Read the model definition and answer for the solid it produces. Units are mm, in the model's axes. Face numbers are marked on the shaded views. A direction names the side the tool comes from. Round coordinates to 2 decimals unless told otherwise and drop trailing zeros. Order: outer loops, then holes, each group sorted by start corner. A loop starts at its lowest first (then second) coordinate and runs counter-clockwise, first axis right, second up. Notation, with made-up numbers: (-37.5, -1) - (-7.5, -1) arc R5 ccw to (-7.5, 4) - close; hole circle Ø8 at (31, 66). An arc over 180 degrees is marked (long way). One line per question, with ' | ' between items. Start each with the question number.
1) For the marked faces 1, 2 and 3, determine the directions among +Z, -Z, +X, -X, +Y, -Y from which every point of the face is accessible in a straight line to the end or side of a thin tool.
2) The part is cut by section D-D, the plane z = -25.5. Give the vertices of the cut face in (x, y) (3 decimals).
3) The part is cut by section C-C, the plane z = 33. Give the vertices of the cut face in (x, y) (3 decimals), plus the area to 3 significant figures.
4) The part is cut by section B-B, the plane x = 0. Give the vertices of the cut face in (y, z) (3 decimals), plus the area to 3 significant figures.
5) Flat-ended cylindrical pins translate along their axes: pin 1 (1 mm diameter, centred on y = 6, z = -29, fed in from +X); pin 2 (1 mm diameter, centred on x = -6, z = -15.5, fed in from -Y); pin 3 (1 mm diameter, centred on y = 0, z = 34, fed in from -X) (3 decimals). Find the tip coordinate at first contact, or state that the pin passes through.
6) The part is cut by section A-A, the plane y = 0. Give the vertices of the cut face in (x, z) (3 decimals).
7) Straight lines are drawn through the part: line 1 (Z direction, x = -0.25, y = 0); line 2 (X direction, y = -0.5, z = 16); line 3 (Y direction, x = 0.25, z = -7). For each, find the intervals that lie inside material, in ascending order. Write a range as from..to.
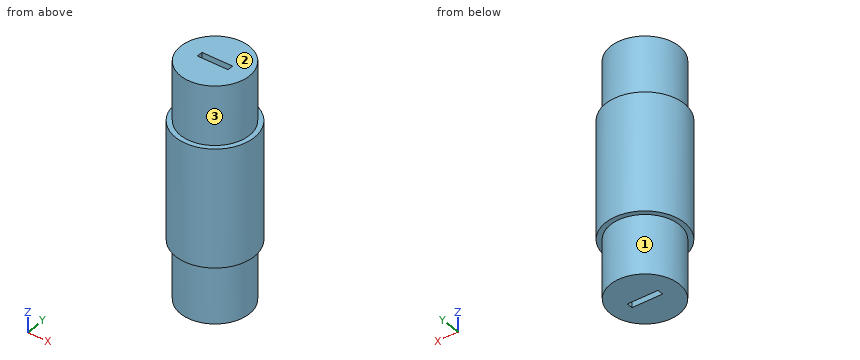
from build123d import *

# Parameters (mm, degrees)
SKETCH1_R                              = 12.7
BASE_EXTRUDE_DEPTH                     = 38.1
SKETCH2_R                              = 12.7
SKETCH2_R_2                            = 11.115
CUT_EXTRUDE1_DEPTH                     = 19.05
SKETCH3_W                              = 10
SKETCH3_H                              = 2
SLOT_FOR_FLAT_BLADE_SCREW_DRIVER_DEPTH = 6


with BuildPart() as part:
    # Sketch1 → Base-Extrude (new body, symmetric)
    with BuildSketch(Plane.XY):
        Circle(SKETCH1_R)
    extrude(amount=BASE_EXTRUDE_DEPTH, both=True)

    # Sketch2 → Cut-Extrude1 (cut)
    with BuildSketch(Plane.XY.offset(38.1)):
        Circle(SKETCH2_R)
        Circle(SKETCH2_R_2, mode=Mode.SUBTRACT)
    cut_extrude1 = extrude(amount=-CUT_EXTRUDE1_DEPTH, mode=Mode.SUBTRACT)

    # Mirror1: Cut-Extrude1 across plane
    add(cut_extrude1.mirror(Plane.XY), mode=Mode.SUBTRACT)

    # Sketch3 → Slot for Flat Blade Screw Driver (cut)
    with BuildSketch(Plane.XY.offset(38.1)):
        Rectangle(SKETCH3_W, SKETCH3_H)
    slot_for_flat_blade_screw_driver = extrude(amount=-SLOT_FOR_FLAT_BLADE_SCREW_DRIVER_DEPTH, mode=Mode.SUBTRACT)

    # Mirror2: Slot for Flat Blade Screw Driver across plane
    add(slot_for_flat_blade_screw_driver.mirror(Plane.XY), mode=Mode.SUBTRACT)


solid = part.part
Values:
1) face 1: -Z | face 2: +Z, +X, -X, +Y, -Y | face 3: +Z
2) outline: circle Ø22.23 at (0, 0)
3) outline: circle Ø22.23 at (0, 0); hole (-5, -1) - (5, -1) - (5, 1) - (-5, 1) - close | area: 368 mm^2
4) outline: (-12.7, -19.05) - (-11.115, -19.05) - (-11.115, -38.1) - (-1, -38.1) - (-1, -32.1) - (1, -32.1) - (1, -38.1) - (11.115, -38.1) - (11.115, -19.05) - (12.7, -19.05) - (12.7, 19.05) - (11.115, 19.05) - (11.115, 38.1) - (1, 38.1) - (1, 32.1) - (-1, 32.1) - (-1, 38.1) - (-11.115, 38.1) - (-11.115, 19.05) - (-12.7, 19.05) - close | area: 1,790 mm^2
5) pin 1: stops at x = 9.66 | pin 2: stops at y = -11.45 | pin 3: stops at x = -11.115
6) outline: (-12.7, -19.05) - (-11.115, -19.05) - (-11.115, -38.1) - (-5, -38.1) - (-5, -32.1) - (5, -32.1) - (5, -38.1) - (11.115, -38.1) - (11.115, -19.05) - (12.7, -19.05) - (12.7, 19.05) - (11.115, 19.05) - (11.115, 38.1) - (5, 38.1) - (5, 32.1) - (-5, 32.1) - (-5, 38.1) - (-11.115, 38.1) - (-11.115, 19.05) - (-12.7, 19.05) - close
7) line 1: z = -32.1..32.1 | line 2: x = -12.69..12.69 | line 3: y = -12.7..12.7
